from build123d import *

# Parameters (mm, degrees)
F0_W     = 5
F0_H     = 90.5
F0_W_2   = 146
F1_DEPTH = 5
F2_W     = 5
F2_H     = 90.5
F3_DEPTH = 5
F4_R     = 1.65
F5_DEPTH = 10.001


with BuildPart() as f1:
    # F0 (on Top) → F1 (new body)
    with BuildSketch(Plane.XY):
        with Locations((75.5, 0)):
            Rectangle(F0_W, F0_H)
        Rectangle(F0_W_2, F0_H)
        with Locations((-75.5, 0)):
            Rectangle(F0_W, F0_H)
    extrude(amount=F1_DEPTH)

    # F2 (on face) → F3 (join)
    with BuildSketch(Plane.XY.offset(5)):
        with Locations((-75.5, 0)):
            Rectangle(F2_W, F2_H)
        with Locations((75.5, 0)):
            Rectangle(F2_W, F2_H)
    extrude(amount=F3_DEPTH)

    # F4 (on face) → F5 (cut, through all)
    with BuildSketch(Plane(origin=(0, 0, 0), x_dir=(1, 0, 0), z_dir=(0, 0, -1))):
        with Locations((-68, 0)):
            Circle(F4_R)
        with Locations((-27, 0)):
            Circle(F4_R)
        with Locations((27, 0)):
            Circle(F4_R)
        with Locations((68, 0)):
            Circle(F4_R)
    extrude(amount=-F5_DEPTH, mode=Mode.SUBTRACT)


solid = f1.part
Read the model definition and answer for the solid it produces. Units are mm, in the model's axes. A direction names the side the tool comes from. Give positions to 0.01 mm unless a question says otherwise; leave off trailing zeros. Write each loop counter-clockwise with the first axis right and the second up, starting at its lowest first coordinate (ties: lowest second). Pieces come first, ordered by that corner, then holes. Notation, with made-up numbers: (19.5, 59.25) - (36.5, 59.25) arc R20 ccw to (36.5, 68.25) - close; hole circle Ø5 at (64.25, -26.5). An arc over 180 degrees is marked (long way). Use CSV: the item, a comma, the result in double quotes. Start each with the question number.
(1) Find section B-B (z = 7). Give the vertices of the cut face in (x, y).
(2) Consider line 1 along X through (y, z) = (0, 3.05); line 2 along X through (y, z) = (-24, 8.75); line 3 along Z through (x, y) = (-51, 6.5). Determine where each line is inside the solid, lowest interval first.
(3) For faces 4 (the cylindrical face through (-28.65, -0.07, 2.46)), 5 (the flat face through (-73, -1, 7)), determine the directions among +Z, -Z, +X, -X, +Y, -Y from which every point of the face is accessible in a straight line to the end or side of a thin tool.
(4) Find section A-A (x = 68). Give the vertices of the cut face in (y, z).
(5) Determine the mould class of faces 1 (the cylindrical face through (66.784, -1.115, 2.465)), 2 (the flat face through (78, -1, 5)), 3 (the flat face through (-1, 45.25, 3)) for opening direction X: +X half, -X half, draft (parallel to the pull), parting line (faces both ways), or undercut.
(6) Given P1, Ø5.5, axis at x = 68, y = 0, coming from the +Z side; P2, Ø3, axis at x = -68, y = 0, coming from the +Z side, each flat-ended and moving along its own axis, determine where each tip first touches the part or whether it passes through.
(7) Find section D-D (y = 19). Give the vertices of the cut face in (x, z).
(8) Find section C-C (y = 0). Give the vertices of the cut face in (x, z).
Findings below:
1,outline,"(-78, -45.25) - (-73, -45.25) - (-73, 45.25) - (-78, 45.25) - close; (73, -45.25) - (78, -45.25) - (78, 45.25) - (73, 45.25) - close"
2,line 1,"-78 to -69.65, -66.35 to -28.65, -25.35 to 25.35, 28.65 to 66.35, 69.65 to 78"
2,line 2,"-78 to -73, 73 to 78"
2,line 3,"0 to 5"
3,face 4,"+Z, -Z"
3,face 5,"+Z, +Y, -Y"
4,outline,"(-45.25, 0) - (-1.65, 0) - (-1.65, 5) - (-45.25, 5) - close; (1.65, 0) - (45.25, 0) - (45.25, 5) - (1.65, 5) - close"
5,face 1,"undercut"
5,face 2,"+X half"
5,face 3,"draft"
6,P1,"z = 5"
6,P2,"through"
7,outline,"(-78, 0) - (78, 0) - (78, 10) - (73, 10) - (73, 5) - (-73, 5) - (-73, 10) - (-78, 10) - close"
8,outline,"(-78, 0) - (-69.65, 0) - (-69.65, 5) - (-73, 5) - (-73, 10) - (-78, 10) - close; (-66.35, 0) - (-28.65, 0) - (-28.65, 5) - (-66.35, 5) - close; (-25.35, 0) - (25.35, 0) - (25.35, 5) - (-25.35, 5) - close; (28.65, 0) - (66.35, 0) - (66.35, 5) - (28.65, 5) - close; (69.65, 0) - (78, 0) - (78, 10) - (73, 10) - (73, 5) - (69.65, 5) - close"
